Here's how the part is built. I have some questions about the finished solid (model axes, mm). A direction names the side the tool comes from. Round coordinates to 2 decimals unless told otherwise and drop trailing zeros. Loops run counter-clockwise (first coordinate to the right, second up) from the corner with the lowest first, then second, coordinate; pieces in that order, holes last. Notation, with made-up numbers: M -34,10 L 24,10 A10 ccw 24,29 Z; hole C 46.5,9.25 d6. An arc over 180 degrees is marked long. One line per question, with ' | ' between items. Start each with the question number.
```python
from build123d import *

# Parameters (mm, degrees)
SKETCH2_W                            = 12.7
SKETCH2_H                            = 12.7
BOSS_EXTRUDE1_DEPTH                  = 38.1
F_1_4_20_THREADED_C_BORE_D           = 6.35
F_1_4_20_THREADED_C_BORE_CBORE_D     = 9.525
F_1_4_20_THREADED_C_BORE_CBORE_DEPTH = 6.35
F_1_4_20_THREADED_HOLE_D             = 6.35


with BuildPart() as part:
    # Sketch2 → Boss-Extrude1 (new, symmetric)
    with BuildSketch(Plane.XY):
        Rectangle(SKETCH2_W, SKETCH2_H)
    extrude(amount=BOSS_EXTRUDE1_DEPTH, both=True)

    # 1/4"-20 threaded C-Bore (through all)
    with Locations(Plane(origin=(0, 6.35, 0), x_dir=(1, 0, 0), z_dir=(0, 1, 0))):
        with Locations((0, 12.7), (0, -12.7)):
            CounterBoreHole(F_1_4_20_THREADED_C_BORE_D / 2, F_1_4_20_THREADED_C_BORE_CBORE_D / 2, F_1_4_20_THREADED_C_BORE_CBORE_DEPTH)

    # 1/4"-20 threaded hole (through all)
    with Locations(Plane(origin=(6.35, 0, 0), x_dir=(0, 0, -1), z_dir=(1, 0, 0))):
        with Locations((-25.4, 0), (0, 0), (25.4, 0)):
            Hole(F_1_4_20_THREADED_HOLE_D / 2)


solid = part.part
```
1) For faces 4 (the face through (3, 3, 9)), 5 (the face through (-0.09, -3.1, -0.69)), which set-ups out of +Z, -Z, +X, -X, +Y, -Y let a thin tool reach every point of the face, with its end or its side?
2) Imagine slicing it at B-B (z = 0). Write out the boundary of the cut face in (x, y) (3 decimals).
3) Imagine slicing it at C-C (y = -5.5). Write out the boundary of the cut face in (x, z) (3 decimals), then the cut area to 3 significant figures.
4) Imagine slicing it at A-A (x = 0). State how many separate pieces and enclosed holes the cut face has, then the cut area to 3 significant figures.
5) I'm going to push a flat-ended pin straight in: pin 1 Ø7.5 at (x, z) = (0, 12.7) entering from +Y. Where does the tip first touch, or does it pass through?
6) We'd pull the mould along Y, two halves only. Please class faces 1 (the face through (-1.03, 3.22, -8.05)), 2 (the face through (-0.09, 0.95, 28.43)), 3 (the face through (0, 6.35, 1)): pulls with the +Y half, pulls with the -Y half, needs draft (parallel to the pull), parting line crosses it, or undercut.
7) Please list where these lines run through material, in increasing order: L1, parallel to Z at x = 0, y = 3.75; L2, parallel to X at y = -4.5, z = -12.7 (3 decimals); L3, parallel to Y at x = -4.25, z = 25.5. Write a range as from..to.
Results are:
1) face 4: +Y | face 5: +X, -X
2) outline: M -6.35,-6.35 L 6.35,-6.35 L 6.35,-3.175 L -6.35,-3.175 Z; M -6.35,3.175 L 6.35,3.175 L 6.35,6.35 L -6.35,6.35 Z
3) outline: M -6.35,-38.1 L 6.35,-38.1 L 6.35,38.1 L -6.35,38.1 Z; hole C 0,-12.7 d6.35; hole C 0,12.7 d6.35 | area: 904 mm²
4) separate pieces: 3 | enclosed holes: 3 | area: 671 mm²
5) pin 1: y = 0
6) face 1: needs draft | face 2: undercut | face 3: pulls with the +Y half
7) L1: -38.1..-17.46, -7.94..7.94, 17.46..38.1 | L2: -6.35..-3.175, 3.175..6.35 | L3: -6.35..-3.17, 3.17..6.35
